Geometry check sheet. Reference: the model listing, model coordinates, mm. Face numbers are marked on the shaded views. A direction names the side the tool comes from. Give positions to 0.01 mm unless a question says otherwise; leave off trailing zeros. Write each loop counter-clockwise with the first axis right and the second up, starting at its lowest first coordinate (ties: lowest second). Pieces come first, ordered by that corner, then holes. Notation, with made-up numbers: (10.5, 62) -> (58.5, 62) arc R8 cw to (58.5, 77) -> close; hole circle Ø10 at (70, -23). An arc over 180 degrees is marked (long way). Write item = value, one per line. Start each with the question number.
1. Cross-section at C-C, the plane x = 61. Record the cut outline in (y, z).
2. Set-up check for the marked faces 1, 2 and 3: record each of +Z, -Z, +X, -X, +Y, -Y from which the full face is reachable in a straight line by a thin tool's end or side.
3. Thickness scan on line 1 along X through (y, z) = (333.93, -12.3) (3 decimals); line 2 along Y through (x, z) = (69.85, 11.5) (3 decimals); line 3 along Z through (x, y) = (3, 42.5). Record the ranges inside material, lowest first.
4. Cross-section at D-D, the plane x = 44.45. Record the cut outline in (y, z) (1 decimal), plus the area to 3 significant figures.
5. Mould release check, pull along Z, two halves, no side actions. Record for the marked faces 4, 5 and 6: pulls with the +Z half, pulls with the -Z half, needs draft (parallel to the pull), parting line crosses it, or undercut.
6. Cross-section at A-A, the plane y = 333.93. State how many separate pieces and enclosed holes the cut face has, plus the area to 3 significant figures.
7. Cross-section at B-B, the plane z = 7.5. Record the cut outline in (x, y).
8. Depth check by flat-ended pin: P1, Ø4, axis at x = 69.85, y = 333.93, coming from the +Z side; P2, Ø8, axis at x = 3.5, z = -6, coming from the -Y side; P3, Ø6.5, axis at y = 90, z = 3, coming from the +X side. Enter the tip coordinate at first touch or a pass-through.
```python
from build123d import *

# Parameters (mm, degrees)
SKETCH1_W           = 25.4
SKETCH1_H           = 25.4
SKETCH1_W_2         = 22.225
SKETCH1_H_2         = 22.225
BOSS_EXTRUDE1_DEPTH = 321.23
SKETCH2_W           = 25.4
SKETCH2_H           = 25.4
SKETCH2_W_2         = 22.225
SKETCH2_H_2         = 22.225
BOSS_EXTRUDE2_DEPTH = 95.25
SKETCH3_R           = 3.175
CUT_EXTRUDE1_DEPTH  = 358.228245524


with BuildPart() as part:
    # Sketch1 → Boss-Extrude1 (new body)
    with BuildSketch(Plane(origin=(0, 0, 0), x_dir=(1, 0, 0), z_dir=(0, 1, 0))):
        Rectangle(SKETCH1_W, SKETCH1_H)
        Rectangle(SKETCH1_W_2, SKETCH1_H_2, mode=Mode.SUBTRACT)
    extrude(amount=BOSS_EXTRUDE1_DEPTH)

    # Sketch2 → Boss-Extrude2 (add)
    with BuildSketch(Plane.ZY.offset(12.7)):
        with Locations((0, 333.93)):
            Rectangle(SKETCH2_W, SKETCH2_H)
        with Locations((0, 333.93)):
            Rectangle(SKETCH2_W_2, SKETCH2_H_2, mode=Mode.SUBTRACT)
    extrude(amount=-BOSS_EXTRUDE2_DEPTH)

    # Sketch3 → Cut-Extrude1 (cut, through all)
    with BuildSketch(Plane.XY.offset(12.7)):
        with Locations((44.45, 333.93)):
            Circle(SKETCH3_R)
        with Locations((69.85, 333.93)):
            Circle(SKETCH3_R)
    extrude(amount=-CUT_EXTRUDE1_DEPTH, mode=Mode.SUBTRACT)


solid = part.part
```
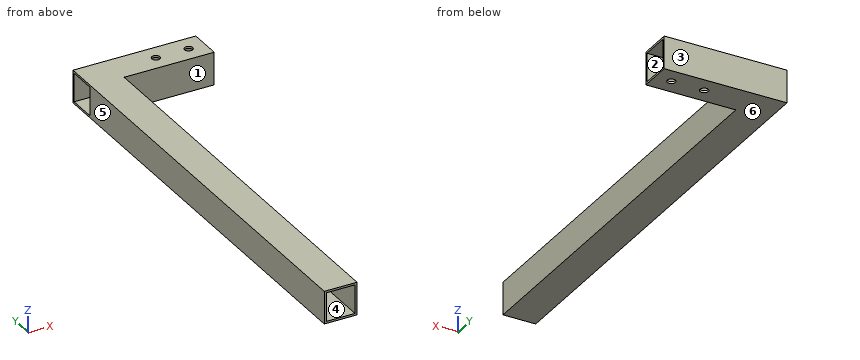
Answers:
q1.outline = (321.23, -12.7) -> (346.63, -12.7) -> (346.63, 12.7) -> (321.23, 12.7) -> close; hole (322.82, -11.11) -> (345.04, -11.11) -> (345.04, 11.11) -> (322.82, 11.11) -> close
q2.face_1 = +Z, -Z, +X, -Y
q2.face_2 = +X, -X
q2.face_3 = +Z, -Z, +X, -X, +Y
q3.line_1 = -12.7 to 41.275, 47.625 to 66.675, 73.025 to 82.55
q3.line_2 = 321.23 to 330.755, 337.105 to 346.63
q3.line_3 = -12.7 to -11.11, 11.11 to 12.7
q4.outline = (321.2, -12.7) -> (330.8, -12.7) -> (330.8, -11.1) -> (322.8, -11.1) -> (322.8, 11.1) -> (330.8, 11.1) -> (330.8, 12.7) -> (321.2, 12.7) -> close; (337.1, -12.7) -> (346.6, -12.7) -> (346.6, 12.7) -> (337.1, 12.7) -> (337.1, 11.1) -> (345, 11.1) -> (345, -11.1) -> (337.1, -11.1) -> close
q4.area = 131 mm^2
q5.face_4 = undercut
q5.face_5 = needs draft
q5.face_6 = pulls with the -Z half
q6.separate_pieces = 6
q6.enclosed_holes = 0
q6.area = 262 mm^2
q7.outline = (-12.7, 0) -> (-11.11, 0) -> (-11.11, 321.23) -> (11.11, 321.23) -> (11.11, 0) -> (12.7, 0) -> (12.7, 321.23) -> (82.55, 321.23) -> (82.55, 322.82) -> (-12.7, 322.82) -> close; (-12.7, 345.04) -> (82.55, 345.04) -> (82.55, 346.63) -> (-12.7, 346.63) -> close
q8.P1 = through
q8.P2 = 321.23
q8.P3 = 12.7
